Drawing for the job (mm, zero at the part's lowest x, y, z). A direction names the side the tool comes from. Round coordinates to 2 decimals unless told otherwise and drop trailing zeros. Write each loop counter-clockwise with the first axis right and the second up, starting at its lowest first coordinate (ties: lowest second). Pieces come first, ordered by that corner, then holes.
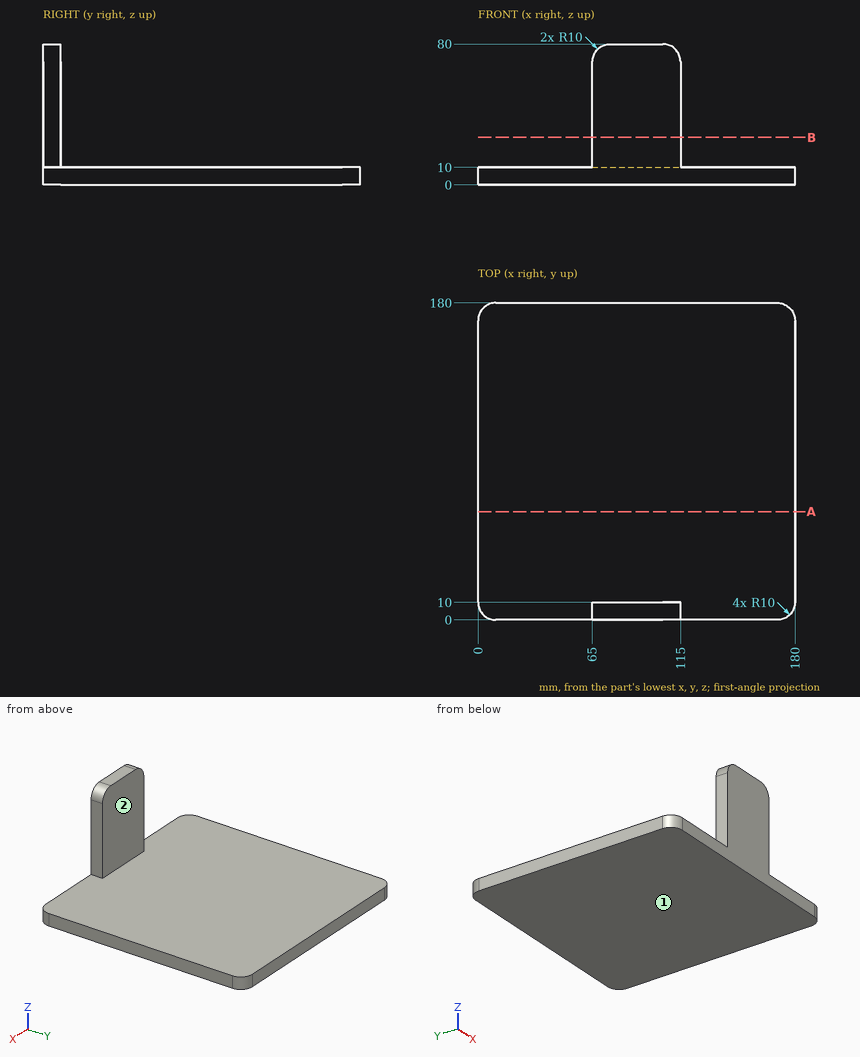
1) Cut at A-A on y = 61.5. List the corners of the cut face in (x, z), and give its area (3 significant figures).
2) Wall check: probe 1 along Z at (x, y) = (85.5, 32). Give the ranges that are in metal, low to high.
3) Cut at B-B on z = 27. List the corners of the cut face in (x, y).
4) Flat gauge pins, fed straight in: pin 1 Ø5 at (x, y) = (103, 134.5) entering from +Z; pin 2 Ø25 at (x, z) = (84.5, 47.5) entering from +Y; pin 3 Ø5 at (y, z) = (4.5, 54.5) entering from -X. Where does each tip first touch, or does it go through?
5) Which spindle directions (+Z, -Z, +X, -X, +Y, -Y) get a long thin tool onto all of the face, cutting with end or side? Do the marked faces 1 and 2. Say none if no direction does.
Result sheet:
1. outline: (0, 0) - (180, 0) - (180, 10) - (0, 10) - close
1. area: 1,800 mm2
2. probe 1: z = 0 to 10
3. outline: (65, 0) - (115, 0) - (115, 10) - (65, 10) - close
4. pin 1: stops at z = 10
4. pin 2: stops at y = 10
4. pin 3: stops at x = 65
5. face 1: -Z, +X, -X, +Y, -Y
5. face 2: +Z, +X, -X, +Y
